Geometry check sheet. Reference: the model listing, model coordinates, mm. A direction names the side the tool comes from. Round coordinates to 2 decimals unless told otherwise and drop trailing zeros. Write each loop counter-clockwise with the first axis right and the second up, starting at its lowest first coordinate (ties: lowest second). Pieces come first, ordered by that corner, then holes.
Item 1: Access from +Z, -Z, +X, -X, +Y, -Y to the whole of each face (thin tool, end or side, straight path). Record for faces 4 (the face through (9.525, 254, 0)), 5 (the face through (-11, 0, 0)).
Item 2: Cross-section at A-A (y = 224). Enter the section's corners in (x, z) (3 decimals).
Item 3: Draft check along X on faces 1 (the face through (-9.525, 254, 0)), 2 (the face through (-11, 514.35, 0)), 3 (the face through (12.7, 254, 0)). Enter one of: pulls with the +X half, pulls with the -X half, needs draft (parallel to the pull), parting line crosses it, or undercut.
Item 4: Scan lines: probe 1 along Y at (x, z) = (0, -11.4); probe 2 along Z at (x, y) = (0.75, 404) (3 decimals); probe 3 along Y at (x, z) = (-2, -10.5). Record each from-to range of solid material in increasing order.
Autodesk Inventor part; units mm, degrees
ref_plane "YZ Plane" through (0, 0, 0) normal (1, 0, 0) x (0, 1, 0)
ref_plane "XZ Plane" through (0, 0, 0) normal (0, 1, 0) x (-1, 0, 0)
ref_plane "XY Plane" through (0, 0, 0) normal (0, 0, 1) x (1, 0, 0)
sketch "Sketch1" plane through (0, 0, 0) normal (0, 1, 0) x (-1, 0, 0)
  line L0 (-12.7, -12.7) -> (12.7, -12.7)
  line L1 (12.7, -12.7) -> (12.7, 12.7)
  line L2 (12.7, 12.7) -> (-12.7, 12.7)
  line L3 (-12.7, 12.7) -> (-12.7, -12.7)
  line L4 (-12.7, -12.7) -> (12.7, 12.7) construction
  line L5 (12.7, -12.7) -> (-12.7, 12.7) construction
  line L6 (9.525, 9.525) -> (9.525, -9.525)
  line L7 (9.525, -9.525) -> (-9.525, -9.525)
  line L8 (-9.525, -9.525) -> (-9.525, 9.525)
  line L9 (-9.525, 9.525) -> (9.525, 9.525)
  point P0 (0, 0)
  dimension "d0" = 25.4
  dimension "d1" = 25.4
  dimension "d2" = 3.175
extrude "Extrusion1" add sketch "Sketch1" along normal blind 514.35
sketch "Sketch4" plane through (-12.7, 0, 12.7) normal (0, 0, 1) x (1, 0, 0)
  line L0 (25.4, 488.95) -> (0, 488.95) construction
  line L1 (0, 488.95) -> (0, 514.35) construction
  line L2 (0, 514.35) -> (25.4, 514.35) construction
  line L3 (25.4, 514.35) -> (25.4, 488.95) construction
  line L4 (25.4, 488.95) -> (0, 514.35) construction
  line L5 (0, 488.95) -> (25.4, 514.35) construction
  circle A0 centre (12.7, 501.65) radius 2.4892
  circle A1 centre (12.7, 463.55) radius 3.2512
  circle A2 centre (12.7, 438.15) radius 3.2512
  point P0 (12.7, 0)
  dimension "d18" = 25.4
  dimension "d19" = 25.4
  dimension "d20" = 4.9784
  dimension "d21" = 6.5024
  dimension "d23" = 25.4
  dimension "d26" = 25.4
extrude "Extrusion4" cut sketch "Sketch4" against normal blind 25.4
sketch "Sketch5" plane through (12.7, 0, 12.7) normal (1, 0, 0) x (0, 0, -1)
  line L0 (0, 0) -> (25.4, 0) construction
  line L1 (3.175, 0) -> (22.225, 0) construction
  line L2 (22.225, 0) -> (22.225, 38.1) construction
  line L3 (22.225, 38.1) -> (3.175, 38.1) construction
  line L4 (3.175, 38.1) -> (3.175, 0) construction
  circle A0 centre (12.7, 44.45) radius 3.2512
  circle A1 centre (12.7, 69.85) radius 3.2512
  circle A2 centre (12.7, 95.25) radius 3.2512
  circle A3 centre (12.7, 336.55) radius 3.2639
  circle A4 centre (12.7, 361.95) radius 3.2639
  circle A5 centre (12.7, 425.45) radius 3.2639
  circle A6 centre (12.7, 450.85) radius 3.2639
  point P0 (12.7, 0)
  point P1 (12.7, 38.1)
  dimension "d27" = 19.05
  dimension "d28" = 38.1
  dimension "d29" = 3.175
  dimension "d30" = 6.5024
  dimension "d31" = 6.35
  dimension "d32" = 25.4
  dimension "d33" = 25.4
  dimension "d38" = 6.5278
  dimension "d39" = 336.55
  dimension "d40" = 25.4
  dimension "d41" = 63.5
  dimension "d42" = 25.4
extrude "Extrusion5" cut sketch "Sketch5" against normal blind 25.4
properties part number "STRU_012_BilletPoleMiddle" material "Aluminum 6061"
Resolved:
1. face 4: +Y, -Y
1. face 5: +Z, -Z, +X, -X, -Y
2. outline: (-12.7, -12.7) - (12.7, -12.7) - (12.7, 12.7) - (-12.7, 12.7) - close; hole (-9.525, -9.525) - (9.525, -9.525) - (9.525, 9.525) - (-9.525, 9.525) - close
3. face 1: undercut
3. face 2: needs draft
3. face 3: pulls with the +X half
4. probe 1: y = 0 to 434.9, 441.4 to 460.3, 466.8 to 499.16, 504.14 to 514.35
4. probe 2: z = -12.7 to -9.525, 9.525 to 12.7
4. probe 3: y = 0 to 435.59, 440.71 to 460.99, 466.11 to 500.17, 503.13 to 514.35
